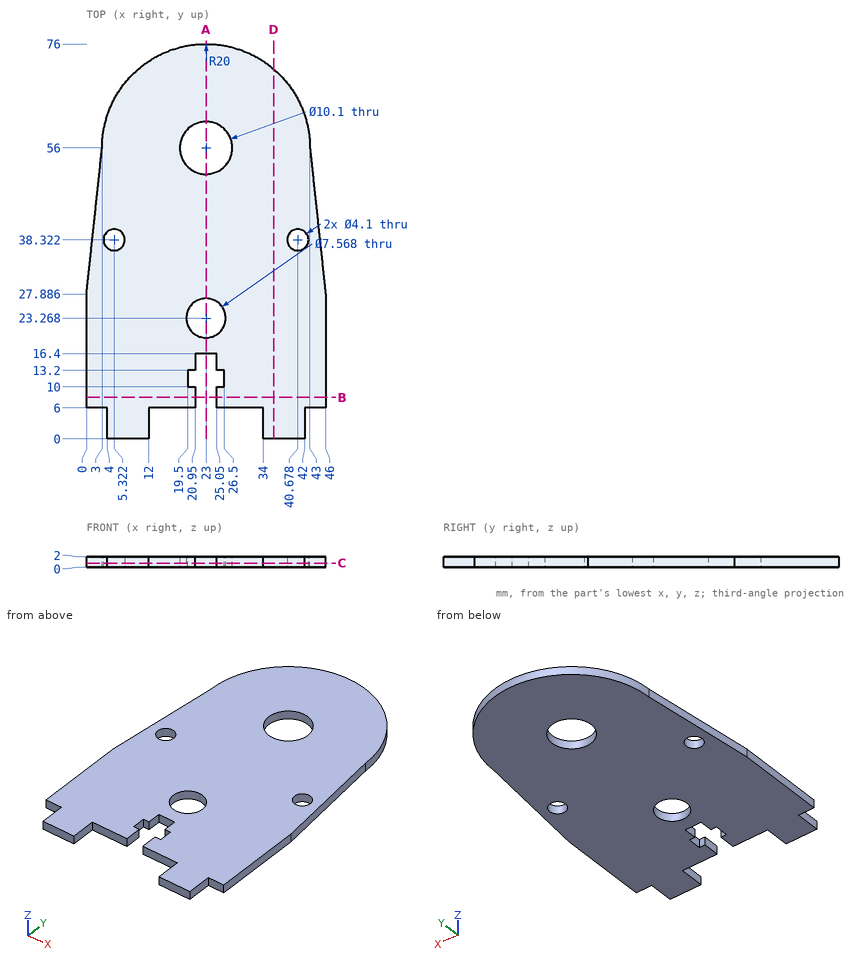
Geometry: see drawing. Coordinates: mm, zero at the bounding-box minimum. Give positions to 0.01 mm unless a question says otherwise; leave off trailing zeros. Loops run counter-clockwise (first coordinate to the right, second up) from the corner with the lowest first, then second, coordinate; pieces in that order, holes last. Notation, with made-up numbers: (4.5, -16.5) - (30.5, -16.5) arc R29 ccw to (30.5, 15.5) - close; hole circle Ø6 at (-24.5, 76.25). An arc over 180 degrees is marked (long way). Use CSV: the item, a comma, the result in double quotes. Start each with the question number.
Item 1: Section A-A on x = 23. Return loops of the section in (y, z).
Item 2: Section D-D on x = 36. Return loops of the section in (y, z).
Item 3: Section C-C on z = 0.8. State how many separate pieces and enclosed holes the cut face has, then the cut area to 3 significant figures.
Item 4: Line query: line 1 (Y direction, x = 23, z = 1.8); line 2 (X direction, y = 12.5, z = 1.4); line 3 (Y direction, x = 20.5, z = 0.5). Output: solid intervals per line, ascending.
Item 5: Contact query for flat-ended pins moving along their axis: P1, Ø0.6, axis at y = 2.5, z = 1, coming from the +X side; P2, Ø0.6, axis at x = 44, z = 1, coming from the -Y side; P3, Ø1, axis at y = 3.5, z = 1, coming from the -X side. Output: stop coordinate, or through.
Item 6: Section B-B on y = 8. Return loops of the section in (x, z).
Ans:
1,outline,"(16.4, 0) - (19.48, 0) - (19.48, 2) - (16.4, 2) - close; (27.05, 0) - (50.95, 0) - (50.95, 2) - (27.05, 2) - close; (61.05, 0) - (76, 0) - (76, 2) - (61.05, 2) - close"
2,outline,"(0, 0) - (71.2, 0) - (71.2, 2) - (0, 2) - close"
3,separate pieces,"1"
3,enclosed holes,"4"
3,area,"2,740 mm2"
4,line 1,"y = 16.4 to 19.48, 27.05 to 50.95, 61.05 to 76"
4,line 2,"x = 0 to 19.5, 26.5 to 46"
4,line 3,"y = 6 to 10, 13.2 to 20.43, 26.11 to 51.61, 60.39 to 75.84"
5,P1,"stops at x = 42"
5,P2,"stops at y = 6"
5,P3,"stops at x = 4"
6,outline,"(0, 0) - (20.95, 0) - (20.95, 2) - (0, 2) - close; (25.05, 0) - (46, 0) - (46, 2) - (25.05, 2) - close"
